from build123d import *

# Parameters (mm, degrees)
PAD_DEPTH = 2


with BuildPart() as part:
    # CopySketch004 → Pad (new body, symmetric)
    with BuildSketch(Plane.XY):
        with BuildLine():
            Line((-96.515385, 5.238812), (-76.217438, 10.233695))
            ThreePointArc((-62.72, 11.87), (-69.518131, 11.459432), (-76.217438, 10.233695))
            Line((-62.72, 11.87), (-42.55212, 11.87))
            Line((-42.55212, 11.87), (21.447979, 11.87))
            ThreePointArc((21.447979, 11.87), (37.950708, 16.369447), (49.885903, 28.622457))
            Line((49.885903, 28.622457), (53.673439, 35.456396))
            Line((53.673439, 35.456396), (100, 35.456396))
            Line((100, 35.456396), (100, 0))
            Line((100, -25.422476), (100, 0))
            Line((53.673439, -25.422476), (100, -25.422476))
            Line((45.758618, -13.259565), (53.673439, -25.422476))
            ThreePointArc((45.758618, -13.259565), (35.575672, -3.722807), (22.130121, 0))
            Line((16, 0), (22.130121, 0))
            Line((16, -10), (16, 0))
            Line((2.15, -10), (16, -10))
            Line((2.15, 1.647389), (2.15, -10))
            Line((-2.15, 1.647389), (2.15, 1.647389))
            Line((-2.15, -10), (-2.15, 1.647389))
            Line((-16, -10), (-2.15, -10))
            Line((-16, 0), (-16, -10))
            Line((-16, 0), (-100, 0.10272))
            ThreePointArc((-96.515385, 5.238812), (-99.243994, 3.339928), (-100, 0.10272))
        make_face()
        with BuildLine():
            ThreePointArc((-73.8787, 7.775189), (-75.3887, 6.265189), (-73.8787, 4.755189))
            Line((-73.8787, 4.755189), (-25.624771, 4.755189))
            ThreePointArc((-25.624771, 4.755189), (-24.114771, 6.265189), (-25.624771, 7.775189))
            Line((-73.8787, 7.775189), (-25.624771, 7.775189))
        make_face(mode=Mode.SUBTRACT)
    extrude(amount=PAD_DEPTH, both=True)


solid = part.part
Model file for the job. Use its own axes, mm. A direction names the side the tool comes from. Coordinates: 2 decimals unless noted, no trailing zeros. Order: outer loops, then holes, each group sorted by start corner. A loop starts at its lowest first (then second) coordinate and runs counter-clockwise, first axis right, second up. Notation, with made-up numbers: M -34,-40 L -9,-40 A31 cw -9,-5 Z; hole C -37.5,2 d4. An arc over 180 degrees is marked long. Return JSON: item names as keys, results as strings.
1. Pull direction X, two halves, no side cores. Call faces 6 (the face through (-50, 7.775, 0)), 7 (the face through (45, 3, -2)), 8 (the face through (49.661, -19.256, 0.028)), 9 (the face through (-2.15, -4, 0)): +X half, -X half, draft (parallel to the pull), parting line (faces both ways), or undercut.
Ans:
{"face 6": "undercut", "face 7": "draft", "face 8": "-X half", "face 9": "undercut"}
2. Flat gauge pins, fed straight in: pin 1 (2 mm diameter, centred on x = -8.5, z = 0, fed in from -Y); pin 2 (1.2 mm diameter, centred on x = -41.5, z = 0, fed in from +Y); pin 3 (2 mm diameter, centred on x = -1, z = -1, fed in from -Y). Where does each tip first touch, or does it go through?
Ans:
{"pin 1": "y = -10", "pin 2": "y = 11.87", "pin 3": "y = 1.65"}
3. Saw through at A-A (z = -0.1). Give the cut face in (x, y), and give its area (3 significant figures).
Ans:
{"outline": "M -100,0.1 L -16,0 L -16,-10 L -2.15,-10 L -2.15,1.65 L 2.15,1.65 L 2.15,-10 L 16,-10 L 16,0 L 22.13,0 A29.2 cw 45.76,-13.26 L 53.67,-25.42 L 100,-25.42 L 100,35.46 L 53.67,35.46 L 49.89,28.62 A32.51 cw 21.45,11.87 L -62.72,11.87 A56.49 ccw -76.22,10.23 L -96.52,5.24 A4.64 ccw Z; hole M -73.88,4.76 L -25.62,4.76 A1.51 ccw -25.62,7.78 L -73.88,7.78 A1.51 ccw Z", "area": "5,100 mm^2"}
4. Tool access for faces 1 (the face through (16, -5, 0)), 2 (the face through (-16, -5, 0)), 3 (the face through (77, -25.422, 0)), 4 (the face through (-50, 4.755, 0)), 5 (the face through (-21, 11.87, 0)): list every direction of +Z, -Z, +X, -X, +Y, -Y with a clear straight run to the whole face (end or side of a thin tool).
Ans:
{"face 1": "+Z, -Z, -Y", "face 2": "+Z, -Z, -X, -Y", "face 3": "+Z, -Z, +X, -X, -Y", "face 4": "+Z, -Z", "face 5": "+Z, -Z, -X, +Y"}
5. Saw through at D-D (x = 39.5). Give the cut face in (y, z).
Ans:
{"outline": "M -6.36,-2 L 17.34,-2 L 17.34,2 L -6.36,2 Z"}
6. Saw through at B-B (x = -66). Give the cut face in (y, z), and give its area (3 significant figures).
Ans:
{"outline": "M 0.06,-2 L 4.76,-2 L 4.76,2 L 0.06,2 Z; M 7.78,-2 L 11.77,-2 L 11.77,2 L 7.78,2 Z", "area": "34.8 mm^2"}
7. Saw through at C-C (y = -4.5). Give the cut face in (x, z), and give its area (3 significant figures).
Ans:
{"outline": "M -16,-2 L -2.15,-2 L -2.15,2 L -16,2 Z; M 2.15,-2 L 16,-2 L 16,2 L 2.15,2 Z; M 36.88,-2 L 100,-2 L 100,2 L 36.88,2 Z", "area": "363 mm^2"}
8. Drill centre lines: probe 1 along X at (y, z) = (1, -1.7); probe 2 along Y at (x, z) = (-45.5, 0.7); probe 3 along X at (y, z) = (-6.5, 1.2). Where is each one in solid material? Low to high.
Ans:
{"probe 1": "-100.04 to -2.15, 2.15 to 100", "probe 2": "0.04 to 4.76, 7.78 to 11.87", "probe 3": "-16 to -2.15, 2.15 to 16, 39.67 to 100"}
